```python
from build123d import *

# Parameters (mm, degrees)
FILLET_1_R = 2


with BuildPart() as part:
    # 草图1 → 旋转1 (revolve)
    with BuildSketch(Plane.XY, mode=Mode.PRIVATE) as revolve_1_sk:
        with BuildLine():
            Line((0, 1), (0, -28.88303688))
            Line((0, -28.88303688), (8, -28.88303688))
            Line((8, -28.88303688), (8, -18.88303688))
            Line((8, -18.88303688), (4, -18.88303688))
            Line((4, -18.88303688), (4, -15.88303688))
            Line((4, -15.88303688), (5, -16.88303688))
            Line((5, -16.88303688), (4, -13.88303688))
            Line((4, -13.88303688), (4, -11.88303688))
            Line((4, -11.88303688), (5, -12.88303688))
            Line((5, -12.88303688), (4, -9.88303688))
            Line((4, -9.88303688), (4, -7.88303688))
            Line((4, -7.88303688), (5, -8.88303688))
            Line((5, -8.88303688), (4, -5.88303688))
            Line((4, -5.88303688), (4, -3.88303688))
            Line((4, -3.88303688), (5, -4.88303688))
            Line((5, -4.88303688), (4, -1.88303688))
            ThreePointArc((4, -1.88303688), (2.465355028, 0.204127172), (0, 1))
        make_face()
    revolve(revolve_1_sk.sketch.rotate(Axis((0, 13.407424858, 0), (0, -1, 0)), 90), axis=Axis((0, 13.407424858, 0), (0, -1, 0)))

    # 圆角1
    fillet_1_edges = [part.edges().sort_by_distance(p)[0] for p in [
        (0, -28.88303688, -8),
    ]]
    fillet(fillet_1_edges, radius=FILLET_1_R)


solid = part.part
```
The model under review builds one solid part; all positions refer to its coordinate system, in mm. A direction names the side the tool comes from. Round coordinates to 2 decimals unless told otherwise and drop trailing zeros. Write each loop counter-clockwise with the first axis right and the second up, starting at its lowest first coordinate (ties: lowest second). Pieces come first, ordered by that corner, then holes. Notation, with made-up numbers: (20, 53.25) - (51, 53.25) arc R32 ccw to (51, 88.25) - close; hole circle Ø6 at (36, 52). An arc over 180 degrees is marked (long way). Use one line per item in the form item = value.
Q1. Draft analysis for pull direction Y (two halves, no side actions). For faces 1 (the flat face through (0, -28.883, 0)), 2 (the cylindrical face through (3.905, -17.362, -0.867)), 3 (the cylindrical face through (7.81, -22.83, -1.73)), state which applies: +Y half, -Y half, draft (parallel to the pull), parting line (faces both ways), or undercut.
Answer key:
face_1 = -Y half
face_2 = undercut
face_3 = draft
Q2. Tool access review of faces 4 (the conical face through (-1.22, -6.03, 3.86)), 5 (the conical face through (3.59, -2.03, 1.87)): name each direction out of +Z, -Z, +X, -X, +Y, -Y from which nothing blocks a thin tool from reaching the whole face with its end or side.
Answer key:
face_4 = none
face_5 = +Y
Q3. Consider section D-D (y = -18.5). State the section outline as (x, z) points.
Answer key:
outline = circle Ø8 at (0, 0)
Q4. Consider section C-C (y = -24). State the section outline as (x, z) points, and give its area (3 significant figures).
Answer key:
outline = circle Ø16 at (0, 0)
area = 201 mm2
Q5. Insertion check: pin 1 Ø2 at (y, z) = (-7, 4.5) entering from -X; pin 2 Ø1 at (x, y) = (4.5, -13) entering from +Z; pin 3 Ø1 at (y, z) = (-10.5, -0.5) entering from -X. Each pin has a flat end and moves straight along its axis. Give the tip position at first contact, or say it passes through.
Answer key:
pin_1 = -2.73
pin_2 = 2.98
pin_3 = -4.35
Q6. For line 1 (Y direction, x = 5.5, z = 1); line 2 (Y direction, x = 3.5, z = 3.25); line 3 (Z direction, x = 2.5, y = -16.25), list the stretches that pass through material, from the lowest coordinate up. Write a range as [from, to].
Answer key:
line_1 = [-28.88, -18.88]
line_2 = [-28.88, -18.88], [-16.66, -16.21], [-12.66, -12.21], [-8.66, -8.21], [-4.66, -4.21]
line_3 = [-4.08, -3.58], [-3.12, 3.12], [3.58, 4.08]
